Read the model definition and answer for the solid it produces. Units are mm, in the model's axes. Round coordinates to 2 decimals unless told otherwise and drop trailing zeros. Write each loop counter-clockwise with the first axis right and the second up, starting at its lowest first coordinate (ties: lowest second). Pieces come first, ordered by that corner, then holes. Notation, with made-up numbers: (16.5, 27) -> (43.5, 27) arc R8 ccw to (43.5, 35) -> close; hole circle Ø2 at (45, 34). An arc over 180 degrees is marked (long way). Return JSON: item names as keys, results as strings. Group by question number.
(1) A cutting plane is placed at C-C on z = 6. State how many separate pieces and enclosed holes the cut face has, then the cut area to 3 significant figures.
(2) Straight lines are drawn through the part: line 1 (Y direction, x = 12.04, z = 10.75); line 2 (Y direction, x = 11.75, z = 11.25); line 3 (Y direction, x = 14.25, z = 8.5). For each, find the intervals that lie inside material, in ascending order.
(3) A cutting plane is placed at B-B on y = 4.5. Give the vertices of the cut face in (x, z).
(4) The mould has two halves that part along Y. Classify faces 1 (the flat face through (-3.2, 3, 10)), 2 (the flat face through (7, 0, 10)), 3 (the cylindrical face through (4.316, 5.593, 10.14)): released by +Y, released by -Y, zero draft, split by the parting line, or undercut.
(5) A cutting plane is placed at A-A on x = 1.88. Give the vertices of the cut face in (y, z).
(6) Given pin 1 (2 mm diameter, centred on x = 4.42, y = 4.8, fed in from -Z); pin 2 (1.3 mm diameter, centred on x = -0.66, y = 4.83, fed in from +Z), each flat-ended and moving along its own axis, determine where each tip first touches the part or whether it passes through.
(7) A cutting plane is placed at D-D on x = 4. Give the vertices of the cut face in (y, z).
```python
from build123d import *

# Parameters (mm, degrees)
BOX_W        = 20.32
BOX_H        = 7
BOX_DEPTH    = 20
SKETCH_R     = 0.8
POCKET_DEPTH = 20


with BuildPart() as part:
    # Box → Box (new body)
    with BuildSketch(Plane(origin=(-3.2, 0, 0), x_dir=(1, 0, 0), z_dir=(0, 0, 1))):
        with Locations((10.16, 3.5)):
            Rectangle(BOX_W, BOX_H)
    extrude(amount=BOX_DEPTH)

    # Sketch → Pocket (cut)
    with BuildSketch(Plane(origin=(-3.2, 0, 20), x_dir=(1, 0, 0), z_dir=(0, 0, 1))):
        with Locations((5.08, 2.26)):
            Circle(SKETCH_R)
        with Locations((7.62, 2.26)):
            Circle(SKETCH_R)
        with Locations((10.16, 2.26)):
            Circle(SKETCH_R)
        with Locations((12.7, 2.26)):
            Circle(SKETCH_R)
        with Locations((15.24, 2.26)):
            Circle(SKETCH_R)
        with Locations((5.08, 4.8)):
            Circle(SKETCH_R)
        with Locations((7.62, 4.8)):
            Circle(SKETCH_R)
        with Locations((10.16, 4.8)):
            Circle(SKETCH_R)
        with Locations((12.7, 4.8)):
            Circle(SKETCH_R)
        with Locations((15.24, 4.8)):
            Circle(SKETCH_R)
        with Locations((2.54, 2.286478)):
            Circle(SKETCH_R)
        with Locations((2.54, 4.826478)):
            Circle(SKETCH_R)
        with Locations((17.78, 2.286478)):
            Circle(SKETCH_R)
    extrude(amount=-POCKET_DEPTH, mode=Mode.SUBTRACT)


solid = part.part
```
Checks:
{
 "1": {"separate pieces": "1", "enclosed holes": "13", "area": "116 mm^2"},
 "2": {"line 1": "y = 0 to 1.46, 3.06 to 4, 5.6 to 7", "line 2": "y = 0 to 1.51, 3.01 to 4.05, 5.55 to 7", "line 3": "y = 0 to 1.56, 3.02 to 7"},
 "3": {"outline": "(-3.2, 0) -> (-1.39, 0) -> (-1.39, 20) -> (-3.2, 20) -> close; (0.07, 0) -> (1.14, 0) -> (1.14, 20) -> (0.07, 20) -> close; (2.62, 0) -> (3.68, 0) -> (3.68, 20) -> (2.62, 20) -> close; (5.16, 0) -> (6.22, 0) -> (6.22, 20) -> (5.16, 20) -> close; (7.7, 0) -> (8.76, 0) -> (8.76, 20) -> (7.7, 20) -> close; (10.24, 0) -> (11.3, 0) -> (11.3, 20) -> (10.24, 20) -> close; (12.78, 0) -> (17.12, 0) -> (17.12, 20) -> (12.78, 20) -> close"},
 "4": {"face 1": "zero draft", "face 2": "released by -Y", "face 3": "undercut"},
 "5": {"outline": "(0, 0) -> (1.46, 0) -> (1.46, 20) -> (0, 20) -> close; (3.06, 0) -> (4, 0) -> (4, 20) -> (3.06, 20) -> close; (5.6, 0) -> (7, 0) -> (7, 20) -> (5.6, 20) -> close"},
 "6": {"pin 1": "stops at z = 0", "pin 2": "passes through"},
 "7": {"outline": "(0, 0) -> (1.58, 0) -> (1.58, 20) -> (0, 20) -> close; (2.94, 0) -> (4.12, 0) -> (4.12, 20) -> (2.94, 20) -> close; (5.48, 0) -> (7, 0) -> (7, 20) -> (5.48, 20) -> close"}
}
